Model file for the job. Use its own axes, mm. Face numbers are marked on the shaded views. A direction names the side the tool comes from. Give positions to 0.01 mm unless a question says otherwise; leave off trailing zeros. Order: outer loops, then holes, each group sorted by start corner. A loop starts at its lowest first (then second) coordinate and runs counter-clockwise, first axis right, second up. Notation, with made-up numbers: (12, -22.75) - (21, -22.75) arc R28 ccw to (21, 4.25) - close; hole circle Ø3 at (-33, -17). An arc over 180 degrees is marked (long way). Use CSV: the item, a comma, the result in double quotes. Start each with the question number.
(1) Band-saw the part on C-C, the plane x = -9. Give the cut face in (y, z) (1 decimal), then the cut area to 3 significant figures.
(2) Drop flat-ended pins along their axis: pin 1 Ø1.8 at (y, z) = (1, 0.5) entering from -X; pin 2 Ø4.5 at (x, y) = (-8.5, 10) entering from +Z; pin 3 Ø6 at (y, z) = (4.5, -3.5) entering from +X. Give the stop position or say it passes through.
(3) Band-saw the part on B-B, the plane y = 0. Give the cut face in (x, z), then the cut area to 3 significant figures.
(4) Probe L1, parallel to Z at x = -11.7, y = 0; L2, parallel to X at y = -4.75, z = 0.5; L3, parallel to Y at x = -9.75, z = 0. List the from-to ranges inside material, lowest first.
(5) Tool access for the marked faces 1, 2 and 3: list every direction of +Z, -Z, +X, -X, +Y, -Y with a clear straight run to the whole face (end or side of a thin tool).
(6) Band-saw the part on D-D, the plane z = 0.75. Give the cut face in (x, y), then the cut area to 3 significant figures.
(7) Band-saw the part on A-A, the plane z = -4.5. Give the cut face in (x, y).
(8) Pull direction X, two halves, no side cores. Call the marked faces 4, 5, 6 and 7: +X half, -X half, draft (parallel to the pull), parting line (faces both ways), or undercut.
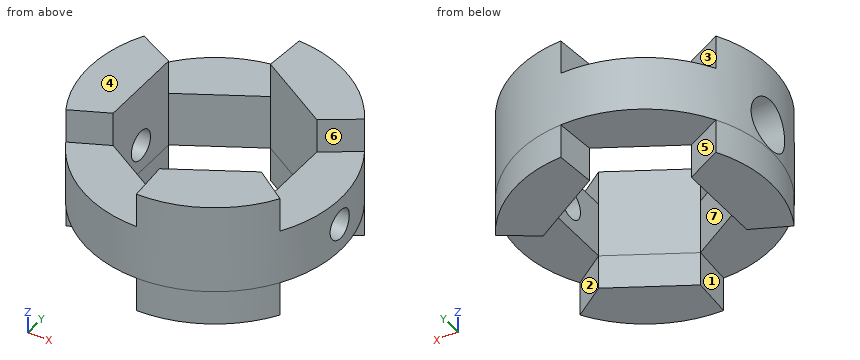
from build123d import *
from build123d.topology import SkipClean

# Parameters (mm, degrees)
SKETCH1_W                = 13.493749999999999
SKETCH1_H                = 9.55675
CUT_EXTRUDE1_DEPTH       = 3.683
CUT_EXTRUDE2_DEPTH       = 3.683
CUT_EXTRUDE3_DEPTH       = 22.342306545626695
BOSS_EXTRUDE1_START      = 3.6830000000000003
BOSS_EXTRUDE1_DEPTH      = 3.6830000000000003
BOSS_EXTRUDE2_DEPTH      = 3.683
BOSS_EXTRUDE3_DEPTH      = 3.683
BOSS_EXTRUDE4_DEPTH      = 3.6830000000000007
M2_CLEARANCE_HOLE1_D     = 2.2606
M2_CLEARANCE_HOLE1_DEPTH = 5.530875
HOLE1_D                  = 3.175
HOLE1_DEPTH              = 26.987525
HOLE1_CBORE_D            = 5.55752
HOLE1_CBORE_DEPTH        = 3.175


with BuildPart() as part:
    # Sketch1 → Revolve1 (revolve)
    with BuildSketch(Plane.XZ, mode=Mode.PRIVATE) as revolve1_sk:
        with Locations((6.746874999999999, 1.8414999999999997)):
            Rectangle(SKETCH1_W, SKETCH1_H)
    revolve(revolve1_sk.sketch.rotate(Axis((0, 0, 6.6198749999999995), (0, 0, -1)), 180), axis=Axis((0, 0, 6.6198749999999995), (0, 0, -1)))

    # Sketch2 → Cut-Extrude1 (cut)
    with BuildSketch(Plane.XY.offset(6.6198749999999995)):
        with BuildLine():
            Line((11.532844262672493, 7.005340268355434), (1.1470002096581853, 6.94e-15))
            Line((1.1470002096581853, 6.94e-15), (11.532844262672493, -7.005340268355431))
            ThreePointArc((11.532844262672493, -7.005340268355431), (13.493749999999999, 1.5e-15), (11.532844262672493, 7.005340268355434))
        make_face()
    extrude(amount=-CUT_EXTRUDE1_DEPTH, mode=Mode.SUBTRACT)

    # Sketch3 → Cut-Extrude2 (cut)
    with BuildSketch(Plane.XY.offset(6.6198749999999995)):
        with BuildLine():
            Line((-0.6429605972199295, -9.714e-14), (0.3003805032135874, 13.490406243541708))
            ThreePointArc((0.3003805032135874, 13.490406243541708), (-13.493749999999999, 1.65e-15), (0.3003805032135965, -13.49040624354171))
            Line((0.3003805032135965, -13.49040624354171), (-0.6429605972199295, -9.714e-14))
        make_face()
    extrude(amount=-CUT_EXTRUDE2_DEPTH, mode=Mode.SUBTRACT)

    # Sketch4 → Cut-Extrude3 (cut, through all)
    with BuildSketch(Plane(origin=(0, 0, -2.936875), x_dir=(-1, 0, 0), z_dir=(0, 0, -1))):
        Polygon((-7.9628999999999985, -4.597382458530073), (0, -9.19476491706014), (7.962900000000002, -4.597382458530068), (7.962900000000002, 4.597382458530077), (-5.2e-15, 9.194764917060152), (-7.962899999999997, 4.5973824585300775), align=None)
    extrude(amount=-CUT_EXTRUDE3_DEPTH, mode=Mode.SUBTRACT)

    # Sketch5 → Boss-Extrude1 (add)
    with BuildSketch(Plane.XY.offset(2.936875).offset(BOSS_EXTRUDE1_START)):
        with BuildLine():
            Line((-11.833224765886177, 6.485065975186222), (-7.962900000000002, 4.597382458530077))
            Line((-7.962900000000002, 4.597382458530077), (-7.962900000000002, -4.597382458530068))
            Line((-7.962900000000002, -4.597382458530068), (-11.833224765886175, -6.485065975186225))
            ThreePointArc((-11.833224765886175, -6.485065975186225), (-13.49375, -1.65e-15), (-11.833224765886177, 6.485065975186222))
        make_face()
    extrude(amount=-BOSS_EXTRUDE1_DEPTH)

    # Sketch6 → Boss-Extrude2 (add)
    with SkipClean():  # the faces are left unmerged after this step: merging them gives an invalid solid
        with BuildSketch(Plane(origin=(0, 0, -2.936875), x_dir=(-1, 0, 0), z_dir=(0, 0, -1))):
            with BuildLine():
                Line((0, 9.194764917060148), (-7.962899999999997, 4.5973824585300775))
                Line((-7.962899999999997, 4.5973824585300775), (-11.53284426267249, 7.005340268355432))
                ThreePointArc((-11.53284426267249, 7.005340268355432), (-6.746874999999971, 11.685930292316284), (-0.30038050321358717, 13.490406243541708))
                Line((-0.30038050321358717, 13.490406243541708), (0, 9.194764917060148))
            make_face()
        extrude(amount=BOSS_EXTRUDE2_DEPTH)

    # Sketch7 → Boss-Extrude3 (add)
    with SkipClean():  # the faces are left unmerged after this step: merging them gives an invalid solid
        with BuildSketch(Plane(origin=(0, 0, -2.936875), x_dir=(-1, 0, 0), z_dir=(0, 0, -1))):
            with BuildLine():
                Line((11.833224765886175, -6.485065975186224), (7.962900000000002, -4.597382458530068))
                Line((7.962900000000002, -4.597382458530068), (7.962900000000002, 4.597382458530077))
                Line((7.962900000000002, 4.597382458530077), (11.833224765886177, 6.485065975186222))
                ThreePointArc((11.833224765886177, 6.485065975186222), (13.49375, 0), (11.833224765886175, -6.485065975186224))
            make_face()
        extrude(amount=BOSS_EXTRUDE3_DEPTH)

    # Sketch8 → Boss-Extrude4 (add)
    with SkipClean():  # the faces are left unmerged after this step: merging them gives an invalid solid
        with BuildSketch(Plane(origin=(0, 0, -2.936875), x_dir=(-1, 0, 0), z_dir=(0, 0, -1))):
            with BuildLine():
                Line((-11.532844262672493, -7.005340268355434), (-7.9628999999999985, -4.597382458530073))
                Line((-7.9628999999999985, -4.597382458530073), (0, -9.19476491706014))
                Line((0, -9.19476491706014), (-0.30038050321359694, -13.49040624354171))
                ThreePointArc((-0.30038050321359694, -13.49040624354171), (-6.746874999999972, -11.685930292316286), (-11.532844262672493, -7.005340268355434))
            make_face()
        extrude(amount=BOSS_EXTRUDE4_DEPTH)

    # M2 Clearance Hole1
    with Locations(Plane.ZY.offset(-7.9628999999999985)):
        with Locations((0, 0)):
            Hole(M2_CLEARANCE_HOLE1_D / 2, depth=M2_CLEARANCE_HOLE1_DEPTH)

    # Hole1
    with Locations(Plane(origin=(-13.49375, 0, 0), x_dir=(0, 0, -1), z_dir=(-1, 0, 0))):
        with Locations((0, 0)):
            CounterBoreHole(HOLE1_D / 2, HOLE1_CBORE_D / 2, HOLE1_CBORE_DEPTH, depth=HOLE1_DEPTH)


solid = part.part
Answer block:
1,outline,"(-10.1, -2.9) - (-5.1, -2.9) - (-5.1, -6.6) - (5.1, -6.6) - (5.1, -2.9) - (10.1, -2.9) - (10.1, 2.9) - (5.1, 2.9) - (5.1, 6.6) - (-5.1, 6.6) - (-5.1, 2.9) - (-10.1, 2.9) - close; hole circle Ø3.2 at (0, 0)"
1,area,"185 mm2"
2,pin 1,"stops at x = -10.32"
2,pin 2,"stops at z = 2.94"
2,pin 3,"stops at x = 13.4"
3,outline,"(-13.49, -6.62) - (-7.96, -6.62) - (-7.96, -1.59) - (-10.32, -1.59) - (-10.32, -2.78) - (-13.49, -2.78) - close; (-13.49, 2.78) - (-10.32, 2.78) - (-10.32, 1.59) - (-7.96, 1.59) - (-7.96, 6.62) - (-13.49, 6.62) - close; (7.96, -2.94) - (13.49, -2.94) - (13.49, -1.59) - (7.96, -1.59) - close; (7.96, 1.59) - (13.49, 1.59) - (13.49, 2.94) - (7.96, 2.94) - close"
3,area,"63.0 mm2"
4,L1,"z = -6.62 to -2.78, 2.78 to 6.62"
4,L2,"x = -12.63 to -7.7, 7.7 to 12.63"
4,L3,"y = -9.33 to -1.59, 1.59 to 9.33"
5,face 1,"-Z, -X, -Y"
5,face 2,"-Z, +X"
5,face 3,"+Z, +Y"
6,outline,"(-13.23, -2.68) arc R13.49 ccw to (13.42, -1.4) - (7.96, -1.4) - (7.96, -4.6) - (0, -9.19) - (-7.96, -4.6) - (-7.96, -1.4) - (-10.32, -1.4) - (-10.32, -2.68) - close; (-13.23, 2.68) - (-10.32, 2.68) - (-10.32, 1.4) - (-7.96, 1.4) - (-7.96, 4.6) - (0, 9.19) - (7.96, 4.6) - (7.96, 1.4) - (13.42, 1.4) arc R13.49 ccw to start"
6,area,"314 mm2"
7,outline,"(-11.83, -6.49) - (-7.96, -4.6) - (-7.96, 4.6) - (-11.83, 6.49) arc R13.49 ccw to start; (0, -9.19) - (0.3, -13.49) arc R13.49 ccw to (11.53, -7.01) - (7.96, -4.6) - close; (0, 9.19) - (7.96, 4.6) - (11.53, 7.01) arc R13.49 ccw to (0.3, 13.49) - close"
8,face 4,"draft"
8,face 5,"undercut"
8,face 6,"+X half"
8,face 7,"undercut"
